from build123d import *

# Parameters (mm, degrees)
SKETCH_1_W          = 30
SKETCH_1_H          = 21
SKETCH_1_R          = 1.5
EXTRUDE_1_DEPTH     = 3
SKETCH_2_W          = 5
SKETCH_2_H          = 15
CUT_EXTRUDE_1_DEPTH = 19.553975315


with BuildPart() as part:
    # 草图1 → 凸台-拉伸1 (new body)
    with BuildSketch(Plane.XY):
        Rectangle(SKETCH_1_W, SKETCH_1_H)
        with Locations((0, 8)):
            Circle(SKETCH_1_R, mode=Mode.SUBTRACT)
        with Locations(Location((0, -8, 0), (0, 0, 180))):
            Circle(SKETCH_1_R, mode=Mode.SUBTRACT)
    extrude(amount=EXTRUDE_1_DEPTH)

    # 草图2 → 切除-拉伸1 (cut, through all)
    with BuildSketch(Plane.XY.offset(3)):
        with Locations((-10, 0)):
            Rectangle(SKETCH_2_W, SKETCH_2_H)
        with Locations((10, 0)):
            Rectangle(SKETCH_2_W, SKETCH_2_H)
    extrude(amount=-CUT_EXTRUDE_1_DEPTH, mode=Mode.SUBTRACT)


solid = part.part
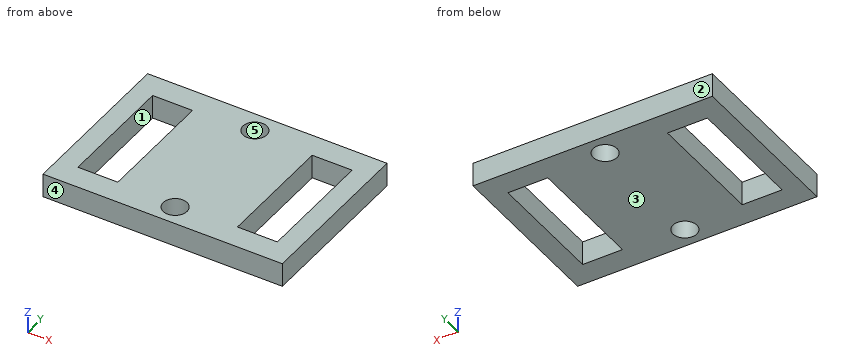
Check sheet for the modelled part. Datum: model origin and axes. Units: mm. Face numbers are marked on the shaded views. A direction names the side the tool comes from. Coordinates: 2 decimals unless noted, no trailing zeros. Loops run counter-clockwise (first coordinate to the right, second up) from the corner with the lowest first, then second, coordinate; pieces in that order, holes last. Notation, with made-up numbers: (74, 88) -> (80, 88) arc R9 ccw to (80, 93) -> close; hole circle Ø7 at (72.5, 18). An arc over 180 degrees is marked (long way). Answer in a Markdown table with one row per item.
1. Sectioned sample at C-C, the plane y = 3.25. Record the boundary of the cut face in (x, z).
Check values:
| item | result |
|---|---|
| outline | (-15, 0) -> (-12.5, 0) -> (-12.5, 3) -> (-15, 3) -> close; (-7.5, 0) -> (7.5, 0) -> (7.5, 3) -> (-7.5, 3) -> close; (12.5, 0) -> (15, 0) -> (15, 3) -> (12.5, 3) -> close |
2. Release check for a two-part mould opening along Y. For the marked faces 3, 4 and 5 record: released by +Y, released by -Y, zero draft, split by the parting line, or undercut.
Check values:
| item | result |
|---|---|
| face 3 | zero draft |
| face 4 | released by -Y |
| face 5 | undercut |
3. Sectioned sample at D-D, the plane z = 2.55. Record the boundary of the cut face in (x, y), then the cut area to 3 significant figures.
Check values:
| item | result |
|---|---|
| outline | (-15, -10.5) -> (15, -10.5) -> (15, 10.5) -> (-15, 10.5) -> close; hole (-12.5, -7.5) -> (-7.5, -7.5) -> (-7.5, 7.5) -> (-12.5, 7.5) -> close; hole circle Ø3 at (0, -8); hole circle Ø3 at (0, 8); hole (7.5, -7.5) -> (12.5, -7.5) -> (12.5, 7.5) -> (7.5, 7.5) -> close |
| area | 466 mm2 |
4. Material ranges on line 1 along Y through (x, z) = (0, 1.55); line 2 along X through (y, z) = (2.75, 1.3); line 3 along X through (y, z) = (-8, 2), recorded low to high. Write a range as [from, to].
Check values:
| item | result |
|---|---|
| line 1 | y = [-10.5, -9.5], [-6.5, 6.5], [9.5, 10.5] |
| line 2 | x = [-15, -12.5], [-7.5, 7.5], [12.5, 15] |
| line 3 | x = [-15, -1.5], [1.5, 15] |
5. Sectioned sample at B-B, the plane x = -10. Record the boundary of the cut face in (y, z).
Check values:
| item | result |
|---|---|
| outline | (-10.5, 0) -> (-7.5, 0) -> (-7.5, 3) -> (-10.5, 3) -> close; (7.5, 0) -> (10.5, 0) -> (10.5, 3) -> (7.5, 3) -> close |
6. Access from +Z, -Z, +X, -X, +Y, -Y to the whole of each face (thin tool, end or side, straight path). Record for the marked faces 1 and 2.
Check values:
| item | result |
|---|---|
| face 1 | +Z, -Z |
| face 2 | +Z, -Z, +X, -X, +Y |
7. Sectioned sample at A-A, the plane x = 0. Record the boundary of the cut face in (y, z).
Check values:
| item | result |
|---|---|
| outline | (-10.5, 0) -> (-9.5, 0) -> (-9.5, 3) -> (-10.5, 3) -> close; (-6.5, 0) -> (6.5, 0) -> (6.5, 3) -> (-6.5, 3) -> close; (9.5, 0) -> (10.5, 0) -> (10.5, 3) -> (9.5, 3) -> close |
